```python
from build123d import *

# Parameters (mm, degrees)
SKETCH1_R           = 1.5000000000000018
SKETCH1_R_2         = 1.5000000000000004
BOSS_EXTRUDE1_DEPTH = 4
BOSS_EXTRUDE2_START = 2
BOSS_EXTRUDE2_DEPTH = 2
BOSS_EXTRUDE3_START = 2
SKETCH3_R           = 1.5000000000000007
SKETCH3_R_2         = 1.500000000000001
BOSS_EXTRUDE3_DEPTH = 2
SKETCH4_R           = 2.921
CUT_EXTRUDE1_DEPTH  = 3.5052
FILLET1_R           = 7.62
SKETCH5_R           = 3.8735000000000004
CUT_EXTRUDE2_DEPTH  = 1.3716


with BuildPart() as part:
    # Sketch1 → Boss-Extrude1 (new body)
    with BuildSketch(Plane(origin=(0, 0, 0), x_dir=(1, 0, 0), z_dir=(0, 1, 0))):
        with BuildLine():
            Line((-3.3528000000000002, -24.130000000000003), (-3.3527999999999993, -6.55871086113727))
            ThreePointArc((-3.3527999999999993, -6.55871086113727), (-7.210684523422123, 1.504654346911835), (-0.45, 7.352241562952077))
            Line((-0.45, 7.352241562952077), (-0.45, 1.325707358356285))
            ThreePointArc((-0.45, 1.325707358356285), (-1.4, 1.7e-16), (-0.45, -1.325707358356285))
            Line((-0.45, -1.325707358356285), (-0.45, -7.780368908234952))
            ThreePointArc((-0.45, -7.780368908234952), (-2.4e-16, -10.3), (0.45000000000000184, -7.780368908234953))
            Line((0.45000000000000184, -7.780368908234953), (0.45000000000000107, -1.3257073583562848))
            ThreePointArc((0.45000000000000107, -1.3257073583562848), (1.4, 0), (0.45000000000000073, 1.3257073583562848))
            Line((0.45000000000000073, 1.3257073583562848), (0.45, 7.352241562952076))
            ThreePointArc((0.45, 7.352241562952076), (7.210684523422123, 1.504654346911832), (3.3527999999999993, -6.55871086113727))
            Line((3.3527999999999993, -6.55871086113727), (3.3528000000000002, -24.130000000000003))
            ThreePointArc((3.3528000000000002, -24.130000000000003), (-6.2e-16, -27.482800000000005), (-3.3528000000000002, -24.130000000000003))
        make_face()
        with Locations(Location((-4.6e-16, -23.9, 0), (0, 0, 270))):
            Circle(SKETCH1_R, mode=Mode.SUBTRACT)
        with Locations(Location((0, -19.9, 0), (0, 0, 270))):
            Circle(SKETCH1_R_2, mode=Mode.SUBTRACT)
    extrude(amount=-BOSS_EXTRUDE1_DEPTH)

    # Sketch2 → Boss-Extrude2 (add)
    with BuildSketch(Plane(origin=(0, 0, 0), x_dir=(1, 0, 0), z_dir=(0, 1, 0)).offset(BOSS_EXTRUDE2_START)):
        with BuildLine():
            Line((-0.44999999999999873, 7.352241562952076), (-0.4499999999999986, 1.325707358356285))
            ThreePointArc((-0.4499999999999986, 1.325707358356285), (-1.3999999999999995, 1.7e-16), (-0.4499999999999986, -1.3257073583562848))
            Line((-0.4499999999999986, -1.3257073583562848), (-0.44999999999999873, -7.352241562952076))
            ThreePointArc((-0.44999999999999873, -7.352241562952076), (-7.366, 9e-16), (-0.44999999999999873, 7.352241562952076))
        make_face()
        with BuildLine():
            Line((0.45, 7.352241562952076), (0.4499999999999999, 1.3257073583562846))
            ThreePointArc((0.4499999999999999, 1.3257073583562846), (1.3999999999999995, 0), (0.4499999999999999, -1.3257073583562846))
            Line((0.4499999999999999, -1.3257073583562846), (0.45, -7.352241562952076))
            ThreePointArc((0.45, -7.352241562952076), (7.366, 0), (0.45, 7.352241562952076))
        make_face()
    extrude(amount=-BOSS_EXTRUDE2_DEPTH)

    # Sketch3 → Boss-Extrude3 (add)
    with BuildSketch(Plane(origin=(0, 0, 0), x_dir=(1, 0, 0), z_dir=(0, 1, 0)).offset(BOSS_EXTRUDE3_START)):
        with BuildLine():
            ThreePointArc((2.611298533252736, -20.95135387488328), (8e-16, -17.085), (-2.6112985332527363, -20.95135387488328))
            ThreePointArc((-2.6112985332527363, -20.95135387488328), (-2.427496854553608, -21.899999999999995), (-2.611298533252737, -22.84864612511671))
            ThreePointArc((-2.611298533252737, -22.84864612511671), (-9.8e-16, -26.715), (2.611298533252737, -22.84864612511671))
            ThreePointArc((2.611298533252737, -22.84864612511671), (2.427496854553609, -21.899999999999995), (2.611298533252736, -20.95135387488328))
        make_face()
        with Locations(Location((0, -19.9, 0), (0, 0, 270))):
            Circle(SKETCH3_R, mode=Mode.SUBTRACT)
        with Locations(Location((-4.6e-16, -23.9, 0), (0, 0, 270))):
            Circle(SKETCH3_R_2, mode=Mode.SUBTRACT)
    extrude(amount=-BOSS_EXTRUDE3_DEPTH)

    # Sketch4 → Cut-Extrude1 (cut)
    with BuildSketch(Plane(origin=(0, 2, 0), x_dir=(1, 0, 0), z_dir=(0, 1, 0))):
        Circle(SKETCH4_R)
    extrude(amount=-CUT_EXTRUDE1_DEPTH, mode=Mode.SUBTRACT)

    # Fillet1
    fillet1_edges = [part.edges().sort_by_distance(p)[0] for p in [
        (-3.3527999999999993, -2, 6.558710861137271),
        (3.352800000000001, -2, 6.55871086113727),
    ]]
    fillet(fillet1_edges, radius=FILLET1_R)

    # Sketch5 → Cut-Extrude2 (cut)
    with BuildSketch(Plane.XZ.offset(4)):
        Circle(SKETCH5_R)
    extrude(amount=-CUT_EXTRUDE2_DEPTH, mode=Mode.SUBTRACT)


solid = part.part
```
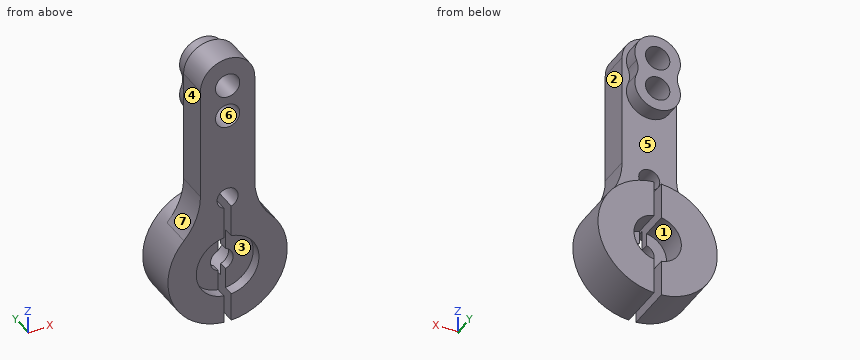
The model under review builds one solid part; all positions refer to its coordinate system, in mm. Face numbers are marked on the shaded views. A direction names the side the tool comes from. Round coordinates to 2 decimals unless told otherwise and drop trailing zeros. Loops run counter-clockwise (first coordinate to the right, second up) from the corner with the lowest first, then second, coordinate; pieces in that order, holes last. Notation, with made-up numbers: (25.25, -8) -> (65.25, -8) arc R20 ccw to (65.25, 1) -> close; hole circle Ø2 at (-22.75, 70). An arc over 180 degrees is marked (long way). Answer as a JSON object with one key per item and string values. Group by question number.
1) Mouldability with a two-part tool opening along Z and no side actions: class the marked faces 4, 5, 6 and 7 as released by +Z, released by -Z, zero draft, split by the parting line, or undercut.
2) We need section A-A on z = 0. Write out the cut boundary in (x, y).
3) For the marked faces 1, 2 and 3, list the 3-axis set-ups (+Z, -Z, +X, -X, +Y, -Y) from which the entire face can be reached by the end or side of a thin tool; tool diameter is ignored.
4) For pin 1 Ø3 at (y, z) = (-0.5, -5.5) entering from +X; pin 2 Ø1 at (x, z) = (-2.5, -1) entering from -Y; pin 3 Ø2 at (x, y) = (-2, 1) entering from -Z, all flat-tipped, find the tip position at first contact; note any pin that passes through.
5) We need section C-C on y = -2.2. Write out the cut boundary in (x, z).
6) We need section B-B on x = 0. Write out the cut boundary in (y, z) (3 decimals).
7) For line 1 (X direction, y = -1.2, z = 19.9); line 2 (Z direction, x = 1, y = -3.1); line 3 (X direction, y = 0.65, z = 0.5), list the stretches that pass through material, from the lowest coordinate up. Write a range as [from, to].
8) We need section D-D on x = -2. Write out the cut boundary in (y, z).
Result set:
{
 "1": {"face 4": "zero draft", "face 5": "undercut", "face 6": "undercut", "face 7": "released by +Z"},
 "2": {"outline": "(-7.37, -4) -> (-3.87, -4) -> (-3.87, -2.63) -> (-1.4, -2.63) -> (-1.4, -1.51) -> (-2.92, -1.51) -> (-2.92, 2) -> (-7.37, 2) -> close; (1.4, -2.63) -> (3.87, -2.63) -> (3.87, -4) -> (7.37, -4) -> (7.37, 2) -> (2.92, 2) -> (2.92, -1.51) -> (1.4, -1.51) -> close"},
 "3": {"face 1": "+Y", "face 2": "+Z, +X, +Y, -Y", "face 3": "-Y"},
 "4": {"pin 1": "x = 6.19", "pin 2": "y = -2.63", "pin 3": "z = -7.3"},
 "5": {"outline": "(-5.39, 5.02) arc R7.37 ccw to (-0.45, -7.35) -> (-0.45, -1.33) arc R1.4 cw to (-0.45, 1.33) -> (-0.45, 7.78) arc R1.3 cw (long way) to (0.45, 7.78) -> (0.45, 1.33) arc R1.4 cw to (0.45, -1.33) -> (0.45, -7.35) arc R7.37 ccw to (5.39, 5.02) arc R7.62 cw to (3.35, 10.21) -> (3.35, 24.13) arc R3.35 ccw to (-3.35, 24.13) -> (-3.35, 10.21) arc R7.62 cw to start; hole circle Ø3 at (0, 19.9); hole circle Ø3 at (0, 23.9)"},
 "6": {"outline": "(-4, 10.3) -> (0, 10.3) -> (0, 17.085) -> (2, 17.085) -> (2, 18.4) -> (-4, 18.4) -> close; (-4, 21.4) -> (2, 21.4) -> (2, 22.4) -> (-4, 22.4) -> close; (-4, 25.4) -> (2, 25.4) -> (2, 26.715) -> (0, 26.715) -> (0, 27.483) -> (-4, 27.483) -> close"},
 "7": {"line 1": "[-3.35, -1.5], [1.5, 3.35]", "line 2": "[-7.3, -3.74], [3.74, 8.17], [9.83, 18.78], [21.02, 22.78], [25.02, 27.33]", "line 3": "[-7.35, -2.88], [2.88, 7.35]"},
 "8": {"outline": "(-4, -7.09) -> (2, -7.09) -> (2, -2.13) -> (-1.51, -2.13) -> (-1.51, 2.13) -> (2, 2.13) -> (2, 7.09) -> (0, 7.09) -> (0, 17.92) -> (2, 17.92) -> (2, 25.88) -> (0, 25.88) -> (0, 26.82) -> (-4, 26.82) -> (-4, 3.32) -> (-2.63, 3.32) -> (-2.63, -3.32) -> (-4, -3.32) -> close"}
}
